Study the drawing (mm; zero at the part's minimum x, y, z) and answer. Round coordinates to 2 decimals unless told otherwise and drop trailing zeros. Order: outer loops, then holes, each group sorted by start corner. A loop starts at its lowest first (then second) coordinate and runs counter-clockwise, first axis right, second up. Notation, with made-up numbers: M 26.5,0.5 L 68.5,0.5 A30 ccw 68.5,35.5 Z; hole C 35,-26.5 d2. An arc over 180 degrees is marked long. Put each result on its own line as item: value. Start each with the question number.
1. The part is cut by section D-D (y = 15.5). Give the vertices of the cut face in (x, z).
2. The part is cut by section B-B (z = 0.85). Count the separate pieces of the cut face and the enclosed holes in it, then the cut area to 3 significant figures.
3. This flat-tipped pin is pushed along its axis until it touches: pin 1 Ø1.5 at (x, y) = (3, 20.525) entering from -Z. Where does it stop, or does it pass through?
4. The part is cut by section C-C (x = 11). Give the vertices of the cut face in (y, z) (1 decimal).
5. Consider line 1 (Y direction, x = 3, z = 0.45) (1 decimal); line 2 (Y direction, x = 2.5, z = 0.35) (1 decimal); line 3 (X direction, y = 11, z = 1) (1 decimal). Determine where each line is inside the solid, lowest interval first.
6. The part is cut by section A-A (x = 21.5). Give the vertices of the cut face in (y, z).
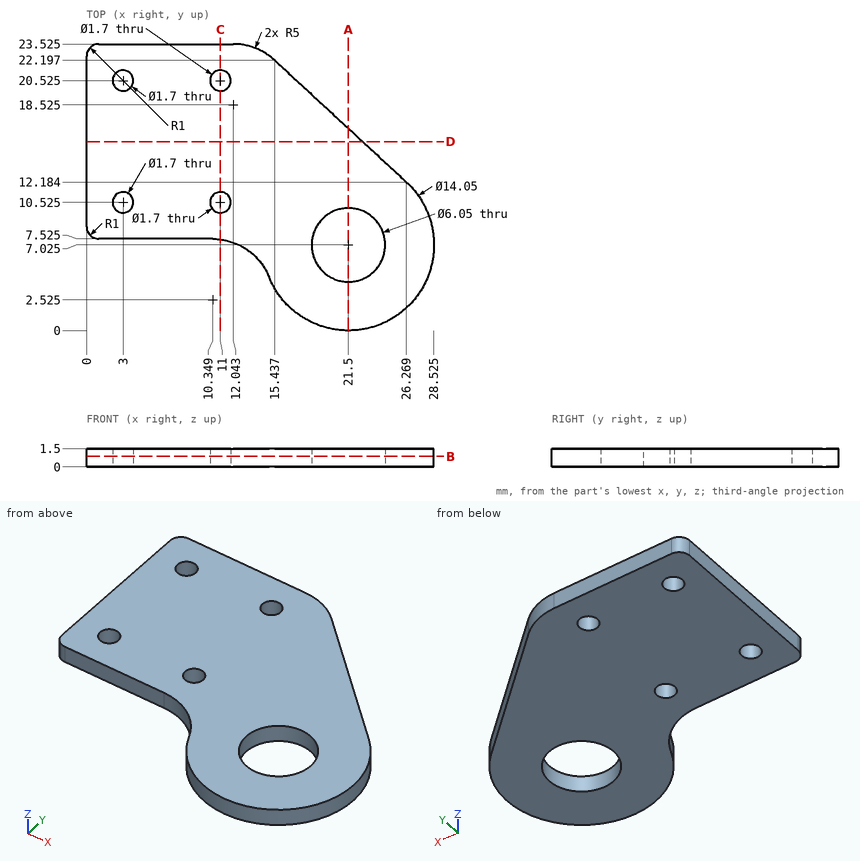
Resolved:
1. outline: M 0,0 L 22.68,0 L 22.68,1.5 L 0,1.5 Z
2. separate pieces: 1
2. enclosed holes: 5
2. area: 406 mm2
3. pin 1: through
4. outline: M 7.5,0 L 9.7,0 L 9.7,1.5 L 7.5,1.5 Z; M 11.4,0 L 19.7,0 L 19.7,1.5 L 11.4,1.5 Z; M 21.4,0 L 23.5,0 L 23.5,1.5 L 21.4,1.5 Z
5. line 1: 7.5 to 9.7, 11.4 to 19.7, 21.4 to 23.5
5. line 2: 7.5 to 9.8, 11.2 to 19.8, 21.2 to 23.5
5. line 3: 0 to 2.3, 3.7 to 10.3, 11.7 to 27.3
6. outline: M 0,0 L 4,0 L 4,1.5 L 0,1.5 Z; M 10.05,0 L 16.59,0 L 16.59,1.5 L 10.05,1.5 Z
